Source: CAD feature listing. Evaluate the final solid. Frame: model axes, mm. A direction names the side the tool comes from. Coordinates: 2 decimals unless noted, no trailing zeros. Order: outer loops, then holes, each group sorted by start corner. A loop starts at its lowest first (then second) coordinate and runs counter-clockwise, first axis right, second up.
Item 1: Section A-A on x = -9.5. Return the cut outline in (y, z).
Item 2: Section B-B on y = 33. Return the cut outline in (x, z).
Item 3: Section D-D on y = 22. Return the cut outline in (x, z), then the cut area to 3 significant figures.
Item 4: Contact query for flat-ended pins moving along their axis: P1, Ø1.2, axis at x = -16.5, y = 6, coming from the +Z side; P2, Ø1.5, axis at x = -18.5, y = 4.5, coming from the +Z side; P3, Ø1, axis at x = -21, z = 18, coming from the +Y side. Output: stop coordinate, or through.
Item 5: Section C-C on z = 20.5. Return the cut outline in (x, y), then the cut area to 3 significant figures.
Item 6: Reachability of faces 1 (the cylindrical face through (-12.312, 36.694, 11.108)), 2 (the cylindrical face through (-12.943, 5.65, 17.911)), 3 (the flat face through (-21, 6, 18.621)), 4 (the flat face through (-14, 37.759, 10)), 5 (the flat face through (-13, 16, 3.221)) from +Z, -Z, +X, -X, +Y, -Y: full face, straight path, thin tool, end or side. Return the list, or none.
Item 7: Ray query, line 1 (Z direction, x = -10.75, y = 19); line 2 (X direction, y = 14, z = 20); line 3 (X direction, y = 16, z = 16.25). Return the intervals inside material, ascending.
Item 8: Mould query, pull axis Y, two halves, no side actions, for faces 6 (the flat face through (-9.006, 21, 17)), 7 (the flat face through (-15, 30.962, 17)), 8 (the cylindrical face through (-17.57, 5.65, 17.91)), 9 (the flat face through (-5, 16, 22.121)). Classes: released by +Y, released by -Y, zero draft, split by the parting line, or undercut.
from build123d import *

# Parameters (mm, degrees)
SKETCH1_W           = 30
SKETCH1_H           = 50
BOSS_EXTRUDE1_DEPTH = 20
SKETCH2_W           = 17.590174706
SKETCH2_H           = 28.27201044
CUT_EXTRUDE1_DEPTH  = 2
BOSS_EXTRUDE2_DEPTH = 7
SKETCH4_R           = 1.783397986
SKETCH4_R_2         = 1.644242452
SKETCH4_R_3         = 1.78177715
BOSS_EXTRUDE3_DEPTH = 2
SKETCH5_R           = 4.074369341
BOSS_EXTRUDE4_DEPTH = 3
SKETCH6_R           = 2.60170509
BOSS_EXTRUDE5_DEPTH = 3
SCALE1_SCALE        = 0.7


with BuildPart() as part:
    # Sketch1 → Boss-Extrude1 (new body)
    with BuildSketch(Plane.XY):
        with Locations((-13.575598108, 16.077578101)):
            Rectangle(SKETCH1_W, SKETCH1_H)
    extrude(amount=BOSS_EXTRUDE1_DEPTH)

    # Sketch2 → Cut-Extrude1 (cut)
    with BuildSketch(Plane.XY.offset(20)):
        with Locations((-16.242560835, 23.231182823)):
            Rectangle(SKETCH2_W, SKETCH2_H)
    extrude(amount=-CUT_EXTRUDE1_DEPTH, mode=Mode.SUBTRACT)

    # Sketch3 → Boss-Extrude2 (add)
    with BuildSketch(Plane.XY.offset(20)):
        Polygon((-4.548684079, 41.077578101), (-5.266390414, 41.077578101), (-5.266390414, -8.922421899), (1.424401892, -8.922421899), (1.424401892, 41.077578101), align=None)
    extrude(amount=BOSS_EXTRUDE2_DEPTH)

    # Sketch4 → Boss-Extrude3 (add)
    with BuildSketch(Plane.XY.offset(20)):
        with Locations((-24.591340484, 1.128947628)):
            Circle(SKETCH4_R)
        with Locations((-18.041639174, 1.128947628)):
            Circle(SKETCH4_R_2)
        with Locations((-11.291658509, 1.128947628)):
            Circle(SKETCH4_R_3)
    extrude(amount=BOSS_EXTRUDE3_DEPTH)

    # Sketch5 → Boss-Extrude4 (add)
    with BuildSketch(Plane(origin=(0, 41.077578101, 0), x_dir=(1, 0, 0), z_dir=(0, 1, 0))):
        with Locations(Location((-14.24940876, -10.110216384, 0), (0, 0, 270))):
            Circle(SKETCH5_R)
    extrude(amount=BOSS_EXTRUDE4_DEPTH)

    # Sketch6 → Boss-Extrude5 (add)
    with BuildSketch(Plane(origin=(0, 44.077578101, 0), x_dir=(1, 0, 0), z_dir=(0, 1, 0))):
        with Locations(Location((-14.364915038, -9.868044196, 0), (0, 0, 270))):
            Circle(SKETCH6_R)
    extrude(amount=BOSS_EXTRUDE5_DEPTH)


with BuildPart() as part_1:
    # Scale1: scaled about (-12.641542426, 16.016298643, 10.736690586)
    add(part.part.scale(SCALE1_SCALE).moved(Location((-3.792462728, 4.804889593, 3.221007176))))


solid = part_1.part
Answer list:
1. outline: (-1.44, 3.22) - (33.56, 3.22) - (33.56, 17.22) - (30.96, 17.22) - (30.96, 15.82) - (11.17, 15.82) - (11.17, 17.22) - (-1.44, 17.22) - close
2. outline: (-23.8, 3.22) - (-2.8, 3.22) - (-2.8, 22.12) - (-7.48, 22.12) - (-7.48, 17.22) - (-23.8, 17.22) - close
3. outline: (-23.8, 3.22) - (-2.8, 3.22) - (-2.8, 22.12) - (-7.48, 22.12) - (-7.48, 17.22) - (-9.01, 17.22) - (-9.01, 15.82) - (-21.32, 15.82) - (-21.32, 17.22) - (-23.8, 17.22) - close
3. area: 300 mm2
4. P1: stops at z = 18.62
4. P2: stops at z = 17.22
4. P3: stops at y = 6.84
5. outline: (-7.48, -1.44) - (-2.8, -1.44) - (-2.8, 33.56) - (-7.48, 33.56) - close
5. area: 164 mm2
6. face 1: +Y
6. face 2: +Z
6. face 3: +Z, -X, +Y, -Y
6. face 4: +Z, -Z, +X, -X, +Y
6. face 5: -Z, +X, -X, +Y, -Y
7. line 1: z = 3.22 to 15.82
7. line 2: x = -7.48 to -2.8
7. line 3: x = -23.8 to -21.32, -9.01 to -2.8
8. face 6: undercut
8. face 7: undercut
8. face 8: split by the parting line
8. face 9: zero draft
